Build history of the part. All positions in model axes, mm. Face numbers are marked on the shaded views. A direction names the side the tool comes from. Give positions to 0.01 mm unless a question says otherwise; leave off trailing zeros. Loops run counter-clockwise (first coordinate to the right, second up) from the corner with the lowest first, then second, coordinate; pieces in that order, holes last.
1) Band-saw the part on D-D on x = -1. List the corners of the cut face in (y, z).
2) Band-saw the part on B-B on x = -10. List the corners of the cut face in (y, z).
3) Band-saw the part on C-C on y = 9. List the corners of the cut face in (x, z), then the cut area to 3 significant figures.
4) Band-saw the part on A-A on z = 6.5. List the corners of the cut face in (x, y).
5) Wall check: line 1 (Z direction, x = 3.5, y = 2.5); line 2 (X direction, y = 12, z = 12); line 3 (Y direction, x = -3, z = 10.5). Give the ranges that are in metal, low to high.
6) 3-axis set-ups, long thin cutter, end or side, ignore diameter. For the marked faces 1, 2 and 3: which of +Z, -Z, +X, -X, +Y, -Y reach the whole face in a straight line?
7) Flat gauge pins, fed straight in: P1, Ø4, axis at x = -9, z = 15, coming from the +Y side; P2, Ø4, axis at y = 5, z = 5.5, coming from the +X side; P3, Ø1.5, axis at x = 0, z = 8.5, coming from the +Y side. Where does each tip first touch, or does it go through?
Autodesk Inventor part; units mm, degrees
ref_plane "YZ Plane" through (0, 0, 0) normal (1, 0, 0) x (0, 1, 0)
ref_plane "XZ Plane" through (0, 0, 0) normal (0, 1, 0) x (-1, 0, 0)
ref_plane "XY Plane" through (0, 0, 0) normal (0, 0, 1) x (1, 0, 0)
sketch "Sketch1" plane through (0, 0, 0) normal (0, 0, 1) x (1, 0, 0)
  line L0 (-37.7472, -6.4088) -> (0.3528, -6.4088)
  line L1 (0.3528, -6.4088) -> (0.3528, 12.6412)
  line L2 (0.3528, 12.6412) -> (-18.6972, 25.3412)
  line L3 (-18.6972, 25.3412) -> (-37.7472, 12.6412)
  line L4 (-37.7472, 12.6412) -> (-37.7472, -6.4088)
  point P0 (0, 0)
  dimension "d0" = 19.05
  dimension "d1" = 19.05
  dimension "d2" = 38.1
  dimension "d3" = 12.7
  dimension "d4" = 19.05
extrude "Extrusion1" add sketch "Sketch1" along normal blind 50.8
sketch "Sketch2" plane through (0.3528, -6.4088, 0) normal (1, 0, 0) x (0, 0, -1)
  line L0 (0, 19.05) -> (-50.8, 19.05)
  line L1 (-38.1, 19.05) -> (-38.1, 0)
  line L2 (0, 0) -> (-50.8, 0)
  line L3 (-38.1, 19.05) -> (-25.4, 28.575)
  line L4 (-25.4, 28.575) -> (-12.7, 19.05)
  line L5 (-12.7, 19.05) -> (-12.7, 0)
  line L6 (-12.7, 0) -> (-38.1, 0)
  line L7 (-50.8, 19.05) -> (-50.8, 0)
  line L8 (0, 0) -> (0, 19.05)
  point P0 (0, 6.4088)
  dimension "d7" = 12.7
  dimension "d8" = 12.7
  dimension "d9" = 9.525
  dimension "d10" = 12.7
extrude "Extrusion2" add sketch "Sketch2" along normal blind 12.7 and the other way blind 17.78 contours L5 L2 L1 L0 | L0 L3 L4
properties part number "Figure 7_28_5"
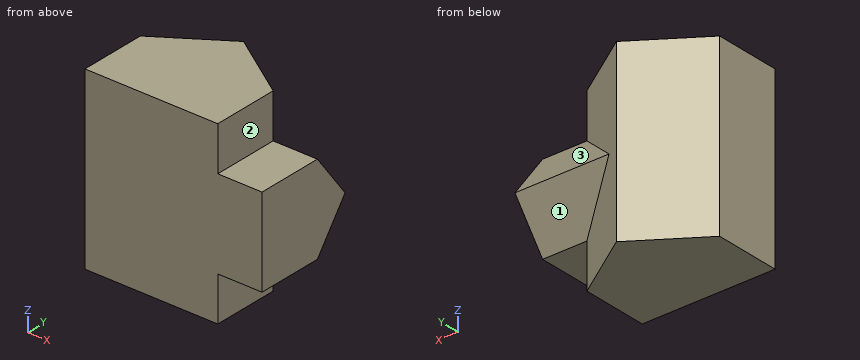
Findings below:
1. outline: (-6.41, 0) - (13.54, 0) - (13.54, 13.9) - (22.17, 25.4) - (13.54, 36.9) - (13.54, 50.8) - (-6.41, 50.8) - close
2. outline: (-6.41, 0) - (19.54, 0) - (19.54, 21.9) - (22.17, 25.4) - (19.54, 28.9) - (19.54, 50.8) - (-6.41, 50.8) - close
3. outline: (-37.75, 0) - (0.35, 0) - (0.35, 12.7) - (13.05, 12.7) - (13.05, 38.1) - (0.35, 38.1) - (0.35, 50.8) - (-37.75, 50.8) - close
3. area: 2,260 mm2
4. outline: (-37.75, -6.41) - (0.35, -6.41) - (0.35, 12.64) - (-18.7, 25.34) - (-37.75, 12.64) - close
5. line 1: z = 12.7 to 38.1
5. line 2: x = -37.75 to 0.35
5. line 3: y = -6.41 to 14.88
6. face 1: -Z, +X, +Y
6. face 2: +Z, +X, +Y, -Y
6. face 3: +Z, +X, +Y
7. P1: stops at y = 20.21
7. P2: stops at x = 0.35
7. P3: stops at y = 13.38
